Read the model definition and answer for the solid it produces. Units are mm, in the model's axes. Face numbers are marked on the shaded views. A direction names the side the tool comes from. Coordinates: 2 decimals unless noted, no trailing zeros. Write each loop counter-clockwise with the first axis right and the second up, starting at its lowest first coordinate (ties: lowest second). Pieces come first, ordered by that corner, then holes. Notation, with made-up numbers: (81, 73.5) -> (124, 73.5) arc R16 ccw to (124, 97.5) -> close; hole circle Ø2 at (63.5, -9.75). An arc over 180 degrees is marked (long way). Return JSON: item names as keys, results as strings.
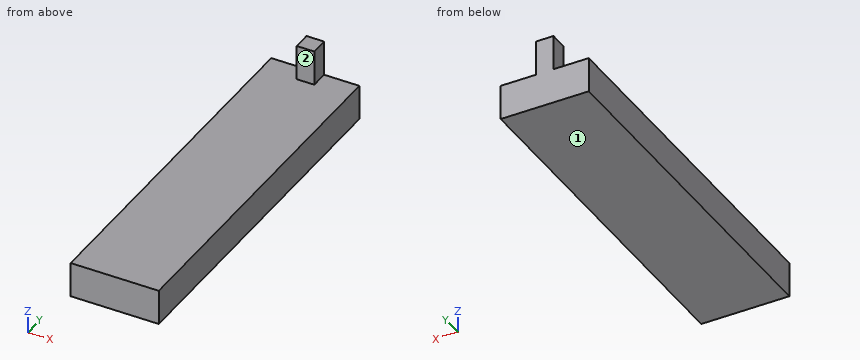
from build123d import *

# Parameters (mm, degrees)
BOSS_EXTRUDE1_DEPTH = 10
SKETCH1_3_W         = 5
SKETCH1_3_H         = 5
BOSS_EXTRUDE2_DEPTH = 20


with BuildPart() as part:
    # Sketch1 → Boss-Extrude1 (new body)
    with BuildSketch(Plane.XY):
        Polygon((-25, 0), (0, 0), (0, 102.5), (-10, 102.5), (-10, 97.5), (-15, 97.5), (-15, 102.5), (-25, 102.5), align=None)
    extrude(amount=BOSS_EXTRUDE1_DEPTH)

    # Sketch1<3> → Boss-Extrude2 (add)
    with BuildSketch(Plane.XY):
        with Locations((-12.5, 100)):
            Rectangle(SKETCH1_3_W, SKETCH1_3_H)
    extrude(amount=BOSS_EXTRUDE2_DEPTH)


solid = part.part
1. Consider L1, parallel to Z at x = -23.25, y = 19.5; L2, parallel to Y at x = -12.5, z = 15.75. Determine where each line is inside the solid, lowest interval first.
Taken from the geometry:
{"L1": "z = 0 to 10", "L2": "y = 97.5 to 102.5"}
2. Flat-ended cylindrical pins translate along their axes: pin 1 Ø4 at (y, z) = (100, 17.5) entering from -X; pin 2 Ø1.5 at (y, z) = (99.5, 12.5) entering from +X; pin 3 Ø12.5 at (x, y) = (-10, 42) entering from +Z; pin 4 Ø1 at (x, z) = (-19.5, 11.5) entering from -Y. Find the tip coordinate at first contact, or state that the pin passes through.
Taken from the geometry:
{"pin 1": "stops at x = -15", "pin 2": "stops at x = -10", "pin 3": "stops at z = 10", "pin 4": "passes through"}
3. A tool of negligible diameter and unlimited length cuts with its end or side. For the marked faces 1 and 2, from which of +Z, -Z, +X, -X, +Y, -Y can it reach the whole face along a straight path? Write none if from no direction.
Taken from the geometry:
{"face 1": "-Z, +X, -X, +Y, -Y", "face 2": "+Z, +X, -X, -Y"}
4. The part is cut by section B-B (x = -4). Determine the outline of the cut face in (y, z), then the cut area to 4 significant figures.
Taken from the geometry:
{"outline": "(0, 0) -> (102.5, 0) -> (102.5, 10) -> (0, 10) -> close", "area": "1,025 mm2"}
5. The part is cut by section A-A (y = 45). Determine the outline of the cut face in (x, z), then the cut area to 3 significant figures.
Taken from the geometry:
{"outline": "(-25, 0) -> (0, 0) -> (0, 10) -> (-25, 10) -> close", "area": "250 mm2"}
